Verification items for the finished model (mm, model axes). Round coordinates to 2 decimals unless told otherwise and drop trailing zeros. Order: outer loops, then holes, each group sorted by start corner. A loop starts at its lowest first (then second) coordinate and runs counter-clockwise, first axis right, second up. Notation, with made-up numbers: (48, 38.25) -> (72, 38.25) arc R9 cw to (72, 54.25) -> close; hole circle Ø2 at (16, 55.25). An arc over 180 degrees is marked (long way). Put each result on its own line as item: value.
```python
from build123d import *

# Parameters (mm, degrees)
SKETCH1_W                  = 12.192
SKETCH1_H                  = 12.192
BOSS_EXTRUDE1_DEPTH        = 52.07
TAP_DRILL_FOR_10_32_TAP1_D = 4.0386
TAP_DRILL_FOR_10_32_TAP2_D = 4.0386


with BuildPart() as part:
    # Sketch1 → Boss-Extrude1 (new, symmetric)
    with BuildSketch(Plane(origin=(0, 0, 0), x_dir=(0, -1, 0), z_dir=(1, 0, 0))):
        Rectangle(SKETCH1_W, SKETCH1_H)
    extrude(amount=BOSS_EXTRUDE1_DEPTH, both=True)

    # Tap Drill for #10-32 Tap1 (through all)
    with Locations(Plane.XY.offset(6.096)):
        with Locations((-45.72, 0), (45.72, 0), (0, 0)):
            Hole(TAP_DRILL_FOR_10_32_TAP1_D / 2)

    # Tap Drill for #10-32 Tap2 (through all)
    with Locations(Plane(origin=(0, 6.096, 0), x_dir=(1, 0, 0), z_dir=(0, 1, 0))):
        with Locations((-30.48, 0), (30.48, 0)):
            Hole(TAP_DRILL_FOR_10_32_TAP2_D / 2)


solid = part.part
```
Item 1: Sectioned sample at A-A, the plane y = 0. Record the boundary of the cut face in (x, z).
Geometry check:
outline: (-52.07, -6.1) -> (-47.74, -6.1) -> (-47.74, 6.1) -> (-52.07, 6.1) -> close; (-43.7, -6.1) -> (-2.02, -6.1) -> (-2.02, 6.1) -> (-43.7, 6.1) -> close; (2.02, -6.1) -> (43.7, -6.1) -> (43.7, 6.1) -> (2.02, 6.1) -> close; (47.74, -6.1) -> (52.07, -6.1) -> (52.07, 6.1) -> (47.74, 6.1) -> close; hole circle Ø4.04 at (-30.48, 0); hole circle Ø4.04 at (30.48, 0)
Item 2: Sectioned sample at C-C, the plane z = 4. Record the boundary of the cut face in (x, y), then the cut area to 3 significant figures.
Geometry check:
outline: (-52.07, -6.1) -> (52.07, -6.1) -> (52.07, 6.1) -> (-52.07, 6.1) -> close; hole circle Ø4.04 at (-45.72, 0); hole circle Ø4.04 at (0, 0); hole circle Ø4.04 at (45.72, 0)
area: 1,230 mm2
Item 3: Material ranges on line 1 along Y through (x, z) = (-45.72, 2.5); line 2 along X through (y, z) = (5.5, 0.25); line 3 along X through (y, z) = (-0.25, 1.25), recorded low to high.
Geometry check:
line 1: -6.1 to -2.02, 2.02 to 6.1
line 2: -52.07 to -32.48, -28.48 to 28.48, 32.48 to 52.07
line 3: -52.07 to -47.72, -43.72 to -32.07, -28.89 to -2, 2 to 28.89, 32.07 to 43.72, 47.72 to 52.07
Item 4: Sectioned sample at B-B, the plane x = -30.48. Record the boundary of the cut face in (y, z), then the cut area to 3 significant figures.
Geometry check:
outline: (-6.1, -6.1) -> (6.1, -6.1) -> (6.1, -2.02) -> (-6.1, -2.02) -> close; (-6.1, 2.02) -> (6.1, 2.02) -> (6.1, 6.1) -> (-6.1, 6.1) -> close
area: 99.4 mm2
Item 5: Sectioned sample at D-D, the plane y = -4.5. Record the boundary of the cut face in (x, z), then the cut area to 3 significant figures.
Geometry check:
outline: (-52.07, -6.1) -> (52.07, -6.1) -> (52.07, 6.1) -> (-52.07, 6.1) -> close; hole circle Ø4.04 at (-30.48, 0); hole circle Ø4.04 at (30.48, 0)
area: 1,240 mm2
Item 6: Depth check by flat-ended pin: pin 1 Ø3.5 at (x, y) = (45.72, 0) entering from -Z; pin 2 Ø5.5 at (x, z) = (30.48, 0) entering from +Y. Enter the tip coordinate at first touch or a pass-through.
Geometry check:
pin 1: through
pin 2: y = 6.1
Item 7: Release check for a two-part mould opening along Z. For faces 1 (the face through (-44.12, -1.23, -0.09)), 2 (the face through (28.554, -0.085, -0.607)), 3 (the face through (1, 3, -6.096)) record: pulls with the +Z half, pulls with the -Z half, needs draft (parallel to the pull), parting line crosses it, or undercut.
Geometry check:
face 1: needs draft
face 2: undercut
face 3: pulls with the -Z half
